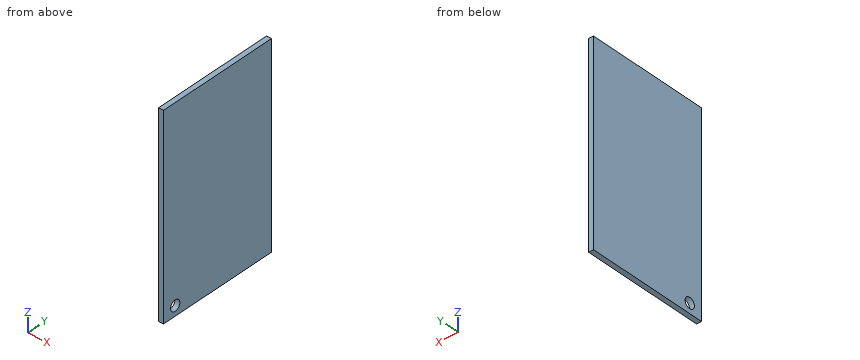
```python
from build123d import *

# Parameters (mm, degrees)
SKETCH_1_W      = 60
SKETCH_1_H      = 37
SKETCH_1_R      = 1.6
EXTRUDE_1_DEPTH = 1.5


with BuildPart() as part:
    # Эскиз1 → Бобышка-Вытянуть1 (new body)
    with BuildSketch(Plane(origin=(0, 0, 0), x_dir=(0, 0, -1), z_dir=(1, 0, 0))):
        with Locations((30, 18.5)):
            Rectangle(SKETCH_1_W, SKETCH_1_H)
        with Locations((3, 4)):
            Circle(SKETCH_1_R, mode=Mode.SUBTRACT)
        with Locations((57, 4)):
            Circle(SKETCH_1_R, mode=Mode.SUBTRACT)
        with Locations((57, 34)):
            Circle(SKETCH_1_R, mode=Mode.SUBTRACT)
        with Locations((3, 34)):
            Circle(SKETCH_1_R, mode=Mode.SUBTRACT)
        with Locations((3, 34)):
            Circle(SKETCH_1_R)
        with Locations((3, 4)):
            Circle(SKETCH_1_R)
        with Locations((57, 34)):
            Circle(SKETCH_1_R)
    extrude(amount=EXTRUDE_1_DEPTH)


solid = part.part
```
Verification items for the finished model (mm, model axes). Round coordinates to 2 decimals unless told otherwise and drop trailing zeros. Order: outer loops, then holes, each group sorted by start corner. A loop starts at its lowest first (then second) coordinate and runs counter-clockwise, first axis right, second up. Notation, with made-up numbers: (-24.5, 76) - (19.5, 76) arc R21 cw to (19.5, 80) - close; hole circle Ø2 at (77.5, 73.25). An arc over 180 degrees is marked (long way). Use CSV: the item, a comma, the result in double quotes. Start each with the question number.
1) Section check B-B, the plane z = -57. Record the cut outline in (x, y), plus the area to 3 significant figures.
2) Section check A-A, the plane y = 4. Record the cut outline in (x, z), plus the area to 3 significant figures.
3) Thickness scan on L1, parallel to Y at x = 0.55, z = -57; L2, parallel to Z at x = 0.3, y = 3.5; L3, parallel to Z at x = 1.4, y = 5. Record the ranges inside material, lowest first.
Answers:
1,outline,"(0, 0) - (1.5, 0) - (1.5, 2.4) - (0, 2.4) - close; (0, 5.6) - (1.5, 5.6) - (1.5, 37) - (0, 37) - close"
1,area,"50.7 mm²"
2,outline,"(0, -60) - (1.5, -60) - (1.5, -58.6) - (0, -58.6) - close; (0, -55.4) - (1.5, -55.4) - (1.5, 0) - (0, 0) - close"
2,area,"85.2 mm²"
3,L1,"y = 0 to 2.4, 5.6 to 37"
3,L2,"z = -60 to -58.52, -55.48 to 0"
3,L3,"z = -60 to -58.25, -55.75 to 0"
